Could you check a few things on this model? Use its own coordinates, in mm. A direction names the side the tool comes from. Round coordinates to 2 decimals unless told otherwise and drop trailing zeros. Write each loop counter-clockwise with the first axis right and the second up, starting at its lowest first coordinate (ties: lowest second). Pieces come first, ordered by that corner, then holes. Notation, with made-up numbers: M 3.5,36 L 12.5,36 A21 ccw 12.5,63 Z; hole C 49.5,-13 d5. An arc over 180 degrees is marked long. One line per question, with ' | ' between items. Start each with the question number.
```python
from build123d import *

# Parameters (mm, degrees)
F1_DEPTH = 19.05
F3_DEPTH = 25.4
F4_D     = 5
F4_DEPTH = 15.6972
F4_TIP   = 1.5021515476


with BuildPart() as f1:
    # F0 (on Top) → F1 (new body)
    with BuildSketch(Plane.XY):
        with BuildLine():
            Line((-22.0673531294, 31.75), (-24.2402065279, 31.75))
            ThreePointArc((-24.2402065279, 31.75), (-39.9455894, 0), (-24.2402065279, -31.75))
            Line((-24.2402065279, -31.75), (-22.0673531294, -31.75))
            Line((-22.0673531294, -31.75), (-22.0673531294, 31.75))
        make_face()
    extrude(amount=F1_DEPTH)

    # F2 (on face) → F3 (cut)
    with BuildSketch(Plane.YZ.offset(-22.0673531294)):
        with BuildLine():
            ThreePointArc((-27.7153407028, 13.9654662391), (-27.8542875294, 11.747165191), (-27.90063, 9.525))
            Line((-27.90063, 9.525), (-22.89937, 9.525))
            ThreePointArc((-22.89937, 9.525), (-22.8573758972, 11.538656851), (-22.7314666127, 13.5488121361))
            ThreePointArc((-22.7314666127, 13.5488121361), (-25.0150766063, 16.2490762326), (-27.7153407028, 13.9654662391))
        make_face()
        with BuildLine():
            Line((-22.89937, 9.525), (-27.90063, 9.525))
            ThreePointArc((-27.90063, 9.525), (-27.8542875294, 7.302834809), (-27.7153407028, 5.0845337609))
            ThreePointArc((-27.7153407028, 5.0845337609), (-25.0150766063, 2.8009237674), (-22.7314666127, 5.5011878639))
            ThreePointArc((-22.7314666127, 5.5011878639), (-22.8573758972, 7.511343149), (-22.89937, 9.525))
        make_face()
    extrude(amount=-F3_DEPTH, mode=Mode.SUBTRACT)

    # F4
    with Locations(Plane.YZ.offset(-22.0673531294)):
        with Locations((25.4, 9.525)):
            Hole(F4_D / 2, depth=F4_DEPTH)
            with Locations((0, 0, -(F4_DEPTH + F4_TIP / 2))):  # 118° drill point
                Cone(0, F4_D / 2, F4_TIP, mode=Mode.SUBTRACT)


solid = f1.part
```
1. If we mould it in two halves opening along Z, with no side actions, what happens to faces 1 (the face through (-26.186, -24.96, 16.244)), 2 (the face through (-26.288, 23.015, 10.276)), 3 (the face through (-22.067, 0, 9)), 4 (the face through (-29, 0, 0))? For each: released by +Z, released by -Z, zero draft, split by the parting line, or undercut.
2. Which directions (+Z, -Z, +X, -X, +Y, -Y) give clear straight access to the entire face, cutting with the end or side of a thin tool? Please do faces 5 (the face through (-29, 0, 19.05)), 6 (the face through (-26.19, -24.23, 3)).
3. Suppose I cut it at A-A (z = 15). Write out the boundary of the cut face in (x, y).
4. Suppose I cut it at B-B (y = -24). Write out the boundary of the cut face in (x, z).
5. Suppose I cut it at C-C (x = -25.75). Write out the boundary of the cut face in (y, z) (3 decimals).
6. I need wall thicknesses on line 1 along Z through (x, y) = (-24.75, 25.4) (3 decimals); line 2 along Y through (x, z) = (-25.25, 11); line 3 along Y through (x, z) = (-25.25, 13.5). Which ranges of each line are inside material? Lowest first, please. Write a range as from..to.
7. Suppose I cut it at D-D (z = 1.5). Write out the boundary of the cut face in (x, y), and give its area (3 significant figures).
8. I'm going to push flat-ended pins straight in: P1, Ø3, axis at y = 13.5, z = 2, coming from the -X side; P2, Ø1.5, axis at y = 3.5, z = 14, coming from the -X side; P3, Ø8, axis at x = -26.5, z = 6, coming from the +Y side; P4, Ø4, axis at y = -20, z = 6, coming from the -X side. Where does each tip first touch, or does it pass through?
Computed:
1) face 1: undercut | face 2: undercut | face 3: zero draft | face 4: released by -Z
2) face 5: +Z, +X, -X, +Y, -Y | face 6: +X, -X
3) outline: M -32.62,-23.05 L -22.07,-23.05 L -22.07,31.75 L -24.24,31.75 A39.95 ccw Z; M -29.07,-27.39 A39.95 ccw -24.24,-31.75 L -22.07,-31.75 L -22.07,-27.39 Z
4) outline: M -31.93,0 L -22.07,0 L -22.07,3.11 L -31.93,3.11 Z; M -31.93,15.94 L -22.07,15.94 L -22.07,19.05 L -31.93,19.05 Z
5) outline: M -30.538,0 L 30.538,0 L 30.538,19.05 L -30.538,19.05 Z; hole M -27.715,5.085 A2.501 ccw -22.731,5.501 A48.299 cw -22.731,13.549 A2.501 ccw -27.715,13.965 A53.301 ccw Z; hole C 25.4,9.525 d5
6) line 1: z = 0..7.025, 12.025..19.05 | line 2: y = -30.95..-27.88, -22.88..23.38, 27.42..30.95 | line 3: y = -30.95..-27.75, -22.74..30.95
7) outline: M -24.24,-31.75 L -22.07,-31.75 L -22.07,31.75 L -24.24,31.75 A39.95 ccw Z | area: 834 mm²
8) P1: stops at x = -38.1 | P2: stops at x = -39.85 | P3: stops at y = 31.75 | P4: stops at x = -35.66
